from build123d import *

# Parameters (mm, degrees)
SKETCH1_W           = 30
SKETCH1_H           = 50
SKETCH1_W_2         = 24
SKETCH1_H_2         = 44
EXTRUDE_THIN1_DEPTH = 50
BOSS_EXTRUDE1_REACH = 78.811
SKETCH2_R           = 5


with BuildPart() as part:
    # Sketch1 → Extrude-Thin1 (new body)
    with BuildSketch(Plane.XY):
        with Locations((15, 25)):
            Rectangle(SKETCH1_W, SKETCH1_H)
        with Locations((15, 25)):
            Rectangle(SKETCH1_W_2, SKETCH1_H_2, mode=Mode.SUBTRACT)
    extrude(amount=EXTRUDE_THIN1_DEPTH)

    # Sketch2 → Boss-Extrude1 (add, up to next)
    with BuildSketch(Plane(origin=(30, 0, 0), x_dir=(0, 0, -1), z_dir=(1, 0, 0)), mode=Mode.PRIVATE) as boss_extrude1_sk1:
        with Locations((-25, 25)):
            Circle(SKETCH2_R)
    boss_extrude1_tool1 = extrude(boss_extrude1_sk1.sketch, amount=-BOSS_EXTRUDE1_REACH, mode=Mode.PRIVATE) - part.part
    add(boss_extrude1_tool1.solids().sort_by_distance((30, 25, 25))[0])


solid = part.part
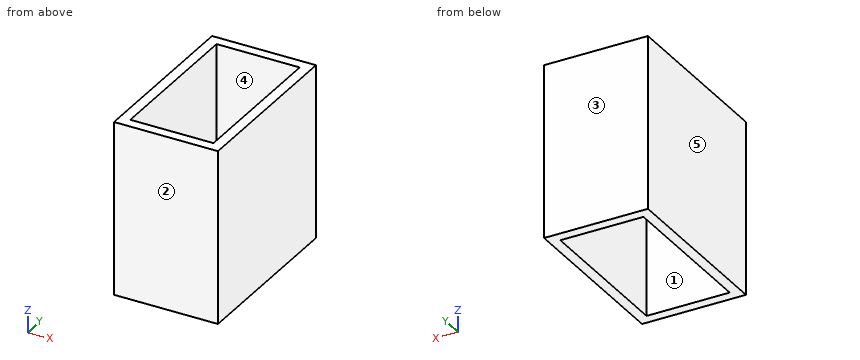
The listing builds one solid part. Answer for the finished solid, in the listing's coordinates (mm). Face numbers are marked on the shaded views. A direction names the side the tool comes from. Round coordinates to 2 decimals unless told otherwise and drop trailing zeros. Write each loop counter-clockwise with the first axis right and the second up, starting at its lowest first coordinate (ties: lowest second). Pieces come first, ordered by that corner, then holes. Notation, with made-up numbers: (-37.75, 30.25) - (-6.75, 30.25) arc R6 ccw to (-6.75, 34.25) - close; hole circle Ø6 at (-35, -34.5). An arc over 180 degrees is marked (long way). Use a Markdown table: item, result. Add a question column.
1. The part is cut by section C-C (x = 21). Write down the section's boundary in (y, z).
2. A tool of negligible diameter and unlimited length cuts with its end or side. For the marked faces 4 and 5, from which of +Z, -Z, +X, -X, +Y, -Y can it reach the whole face along a straight path? Write none if from no direction.
3. The part is cut by section B-B (z = 25). Write down the section's boundary in (x, y), and give its area (3 significant figures).
4. The part is cut by section A-A (y = 14). Write down the section's boundary in (x, z), and give its area (3 significant figures).
5. Consider line 1 (Y direction, x = 26.5, z = 37.5); line 2 (X direction, y = 32.5, z = 40); line 3 (Y direction, x = 16, z = 28). Determine where each line is inside the solid, lowest interval first.
6. For a pull along Y with two mould halves and no side action, classify the marked faces 1, 2 and 3 as +Y half, -Y half, draft (parallel to the pull), parting line (faces both ways), or undercut.
7. The part is cut by section D-D (z = 36). Write down the section's boundary in (x, y), and give its area (3 significant figures).
Reported:
| question | item | result |
|---|---|---|
| 1 | outline | (0, 0) - (3, 0) - (3, 50) - (0, 50) - close; circle Ø10 at (25, 25); (47, 0) - (50, 0) - (50, 50) - (47, 50) - close |
| 2 | face 4 | +Z, -Z |
| 2 | face 5 | +Z, -Z, -X, +Y, -Y |
| 3 | outline | (0, 0) - (30, 0) - (30, 50) - (0, 50) - close; hole (3, 3) - (27, 3) - (27, 20) - (3, 20) - close; hole (3, 30) - (27, 30) - (27, 47) - (3, 47) - close |
| 3 | area | 684 mm^2 |
| 4 | outline | (0, 0) - (3, 0) - (3, 50) - (0, 50) - close; (27, 0) - (30, 0) - (30, 50) - (27, 50) - close |
| 4 | area | 300 mm^2 |
| 5 | line 1 | 0 to 3, 47 to 50 |
| 5 | line 2 | 0 to 3, 27 to 30 |
| 5 | line 3 | 0 to 3, 21 to 29, 47 to 50 |
| 6 | face 1 | undercut |
| 6 | face 2 | -Y half |
| 6 | face 3 | +Y half |
| 7 | outline | (0, 0) - (30, 0) - (30, 50) - (0, 50) - close; hole (3, 3) - (27, 3) - (27, 47) - (3, 47) - close |
| 7 | area | 444 mm^2 |
